```python
from build123d import *

# Parameters (mm, degrees)
EXTRUDE_1_DEPTH     = 9
SKETCH_2_R          = 12.5
CUT_EXTRUDE_1_DEPTH = 10
SKETCH_3_R          = 13.5
SKETCH_3_R_2        = 12.5
EXTRUDE_2_DEPTH     = 3
SKETCH_4_R          = 13.5
SKETCH_4_R_2        = 12.5
EXTRUDE_3_DEPTH     = 1
SKETCH_5_R          = 9.5
CUT_EXTRUDE_2_DEPTH = 11


with BuildPart() as part:
    # 스케치1 → 보스-돌출1 (new body)
    with BuildSketch(Plane(origin=(0, 0, 0), x_dir=(1, 0, 0), z_dir=(0, 1, 0))):
        with BuildLine():
            Line((-12.5, -260), (-12.5, -12.247448714))
            ThreePointArc((-12.5, -12.247448714), (0, 17.5), (12.5, -12.247448714))
            Line((12.5, -12.247448714), (12.5, -260))
            ThreePointArc((12.5, -260), (0, -272.5), (-12.5, -260))
        make_face()
    extrude(amount=EXTRUDE_1_DEPTH)

    # 스케치2 → 컷-돌출1 (cut, through all)
    with BuildSketch(Plane(origin=(0, 9, 0), x_dir=(1, 0, 0), z_dir=(0, 1, 0))):
        Circle(SKETCH_2_R)
    extrude(amount=-CUT_EXTRUDE_1_DEPTH, mode=Mode.SUBTRACT)

    # 스케치3 → 보스-돌출2 (add)
    with BuildSketch(Plane(origin=(0, 9, 0), x_dir=(1, 0, 0), z_dir=(0, 1, 0))):
        Circle(SKETCH_3_R)
        Circle(SKETCH_3_R_2, mode=Mode.SUBTRACT)
    extrude(amount=EXTRUDE_2_DEPTH)

    # 스케치4 → 보스-돌출3 (add)
    with BuildSketch(Plane.XZ):
        Circle(SKETCH_4_R)
        Circle(SKETCH_4_R_2, mode=Mode.SUBTRACT)
    extrude(amount=EXTRUDE_3_DEPTH)

    # 스케치5 → 컷-돌출2 (cut, through all)
    with BuildSketch(Plane(origin=(0, 9, 0), x_dir=(1, 0, 0), z_dir=(0, 1, 0))):
        with Locations((0, -250)):
            Circle(SKETCH_5_R)
    extrude(amount=-CUT_EXTRUDE_2_DEPTH, mode=Mode.SUBTRACT)


solid = part.part
```
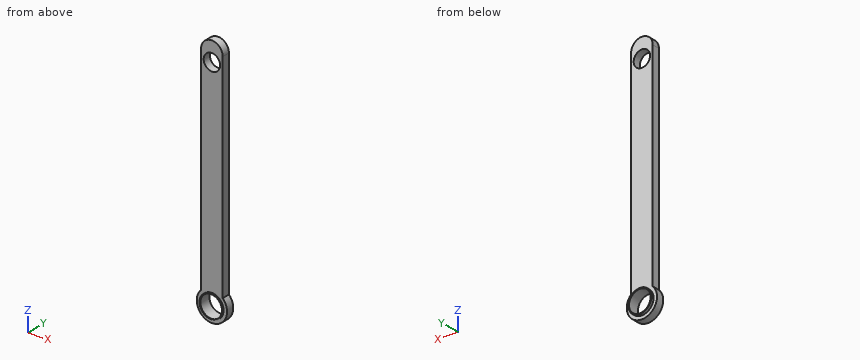
Source: CAD feature listing. Evaluate the final solid. Frame: model axes, mm. Coordinates: 2 decimals unless noted, no trailing zeros. Loops run counter-clockwise (first coordinate to the right, second up) from the corner with the lowest first, then second, coordinate; pieces in that order, holes last. Notation, with made-up numbers: M -26,1 L -19,1 A18 ccw -19,29 Z; hole C 9,-20 d4. An arc over 180 degrees is marked long. Use a Markdown table: item, result. Add a question column.
Q1. Section query C-C, the plane y = 6.75. Return loops of the section in (x, z), and give its area (3 significant figures).
Q2. Material intervals for L1, parallel to Z at x = 0, y = 7.25; L2, parallel to Z at x = -3, y = 0.25; L3, parallel to X at y = 4.25, z = 0, sorted ascending.
Q3. Section query D-D, the plane z = 0. Return loops of the section in (x, y), and give its area (3 significant figures).
Q4. Section query B-B, the plane x = 0. Return loops of the section in (y, z).
Q5. Section query A-A, the plane z = 250. Return loops of the section in (x, y), and give its area (3 significant figures).
Q6. First-contact query: pin 1 (10.5 mm diameter, centred on x = -2, z = 118.5, fed in from -Y); pin 2 (1.5 mm diameter, centred on y = 9.5, z = 217, fed in from -X); pin 3 (3 mm diameter, centred on x = 1.5, y = 1.5, fed in from -Z); pin 4 (1.5 mm diameter, centred on x = -10.5, y = 6, fed in from -Z). Flat tips, straight axial feed; report the tip coordinate or a pass-through.
Result:
| question | item | result |
|---|---|---|
| 1 | outline | M -12.5,12.25 A17.5 ccw long 12.5,12.25 L 12.5,260 A12.5 ccw -12.5,260 Z; hole C 0,0 d25; hole C 0,250 d19 |
| 1 | area | 6,540 mm2 |
| 2 | L1 | z = -17.5 to -12.5, 12.5 to 240.5, 259.5 to 272.5 |
| 2 | L2 | z = -17.24 to -12.13, 12.13 to 240.99, 259.01 to 272.13 |
| 2 | L3 | x = -17.5 to -12.5, 12.5 to 17.5 |
| 3 | outline | M -17.5,0 L -13.5,0 L -13.5,-1 L -12.5,-1 L -12.5,12 L -13.5,12 L -13.5,9 L -17.5,9 Z; M 12.5,-1 L 13.5,-1 L 13.5,0 L 17.5,0 L 17.5,9 L 13.5,9 L 13.5,12 L 12.5,12 Z |
| 3 | area | 98.0 mm2 |
| 4 | outline | M -1,-13.5 L 0,-13.5 L 0,-17.5 L 9,-17.5 L 9,-13.5 L 12,-13.5 L 12,-12.5 L -1,-12.5 Z; M -1,12.5 L 12,12.5 L 12,13.5 L 9,13.5 L 9,240.5 L 0,240.5 L 0,13.5 L -1,13.5 Z; M 0,259.5 L 9,259.5 L 9,272.5 L 0,272.5 Z |
| 5 | outline | M -12.5,0 L -9.5,0 L -9.5,9 L -12.5,9 Z; M 9.5,0 L 12.5,0 L 12.5,9 L 9.5,9 Z |
| 5 | area | 54.0 mm2 |
| 6 | pin 1 | stops at y = 0 |
| 6 | pin 2 | stops at x = -12.5 |
| 6 | pin 3 | stops at z = -17.5 |
| 6 | pin 4 | stops at z = -14.53 |
